from build123d import *

# Parameters (mm, degrees)
SKETCH048_W     = 16
SKETCH048_H     = 8
PAD027_DEPTH    = 12
SKETCH049_W     = 7.6
SKETCH049_H     = 8
POCKET017_DEPTH = 7
SKETCH050_W     = 3
SKETCH050_H     = 6
POCKET018_DEPTH = 16.001
SKETCH060_W     = 3.4
SKETCH060_H     = 2
PAD032_DEPTH    = 9


with BuildPart() as part:
    # Sketch048 → Pad027 (new body)
    with BuildSketch(Plane.YZ):
        with Locations((0, 4)):
            Rectangle(SKETCH048_W, SKETCH048_H)
    extrude(amount=PAD027_DEPTH)

    # Sketch049 (on Face6 of Pad027) → Pocket017 (cut)
    with BuildSketch(Plane.YZ.offset(12)):
        with Locations((0, 4)):
            Rectangle(SKETCH049_W, SKETCH049_H)
    extrude(amount=-POCKET017_DEPTH, mode=Mode.SUBTRACT)

    # Sketch050 (on Face9 of Pocket017) → Pocket018 (cut, through all)
    with BuildSketch(Plane(origin=(0, -8, 0), x_dir=(0, 0, -1), z_dir=(0, -1, 0))):
        with Locations((-1.5, 9)):
            Rectangle(SKETCH050_W, SKETCH050_H)
    extrude(amount=-POCKET018_DEPTH, mode=Mode.SUBTRACT)

    # Sketch060 (on Face5 of Pocket018) → Pad032 (join)
    with BuildSketch(Plane(origin=(0, 3.8, 0), x_dir=(0, 0, -1), z_dir=(0, -1, 0))):
        with Locations((-6.3, 11)):
            Rectangle(SKETCH060_W, SKETCH060_H)
    extrude(amount=PAD032_DEPTH)


with BuildPart() as part_1:
    # Body005 placement: moved
    add(part.part.moved(Location((-45.5, -30.1, 10.6))))


solid = part_1.part
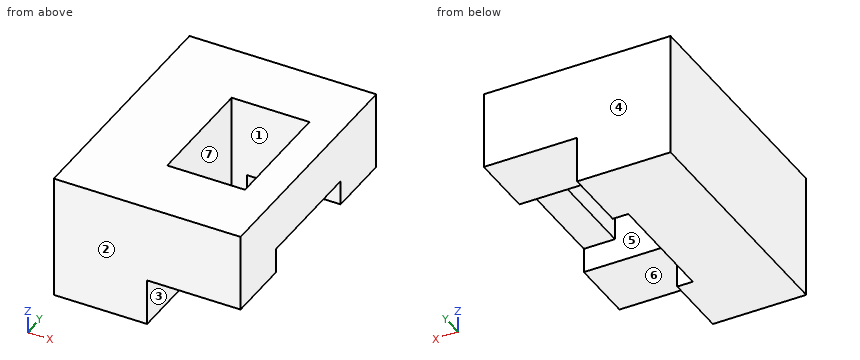
Input: part model. Units: mm. Frame: model coordinates. Face numbers are marked on the shaded views. A direction names the side the tool comes from. Give positions to 0.01 mm unless a question says otherwise; leave off trailing zeros. Loops run counter-clockwise (first coordinate to the right, second up) from the corner with the lowest first, then second, coordinate; pieces in that order, holes last. Notation, with made-up numbers: M -16,-35 L -4,-35 A15 ccw -4,-12 Z; hole C 64,81 d8. An arc over 180 degrees is marked long. Use one line per item in the form item = value.
1. Reachability of the marked faces 5, 6 and 7 from +Z, -Z, +X, -X, +Y, -Y: full face, straight path, thin tool, end or side. Return the list, or none.
Numbers:
face_5 = -Z
face_6 = -Z, +X, +Y, -Y
face_7 = +Z, -Z
2. Line query: L1, parallel to X at y = -29.75, z = 16; L2, parallel to Y at x = -36.75, z = 17; L3, parallel to Z at x = -33.75, y = -25.5. Output: solid intervals per line, ascending.
Numbers:
L1 = -45.5 to -40.5, -35.5 to -33.5
L2 = -38.1 to -33.9, -26.3 to -22.1
L3 = 13.6 to 18.6
3. Section query C-C, the plane y = -26.75. Return the cut outline in (x, z).
Numbers:
outline = M -45.5,10.6 L -40.5,10.6 L -40.5,18.6 L -45.5,18.6 Z; M -35.5,15.2 L -33.5,15.2 L -33.5,18.6 L -35.5,18.6 Z
4. Pull-direction query (Y, two-part tool) for the marked faces 1, 2, 3 and 4; classes: released by +Y, released by -Y, zero draft, split by the parting line, or undercut.
Numbers:
face_1 = undercut
face_2 = released by -Y
face_3 = zero draft
face_4 = released by +Y
5. First-contact query: pin 1 (1 mm diameter, centred on x = -34, y = -29, fed in from -Z); pin 2 (3 mm diameter, centred on y = -28, z = 11.5, fed in from +X); pin 3 (1.3 mm diameter, centred on x = -36, y = -35.5, fed in from -Z). Flat tips, straight axial feed; report the tip coordinate or a pass-through.
Numbers:
pin_1 = 15.2
pin_2 = -40.5
pin_3 = 13.6
6. Section query D-D, the plane z = 15. Return the cut outline in (x, y).
Numbers:
outline = M -45.5,-38.1 L -33.5,-38.1 L -33.5,-33.9 L -40.5,-33.9 L -40.5,-26.3 L -33.5,-26.3 L -33.5,-22.1 L -45.5,-22.1 Z
7. Section query B-B, the plane x = -36. Return the cut outline in (y, z), and give its area (3 significant figures).
Numbers:
outline = M -38.1,13.6 L -33.9,13.6 L -33.9,18.6 L -38.1,18.6 Z; M -26.3,13.6 L -22.1,13.6 L -22.1,18.6 L -26.3,18.6 Z
area = 42.0 mm²
8. Section query A-A, the plane z = 17. Return the cut outline in (x, y).
Numbers:
outline = M -45.5,-38.1 L -33.5,-38.1 L -33.5,-22.1 L -45.5,-22.1 Z; hole M -40.5,-33.9 L -35.5,-33.9 L -35.5,-26.3 L -40.5,-26.3 Z
